Autodesk Inventor part; units mm, degrees
ref_plane "Work Plane1" through (-12.7, 65.9911, 38.1) normal (0, 0.866, 0.5) x (1, 0, 0)
ref_plane "YZ Plane" through (0, 0, 0) normal (1, 0, 0) x (0, 1, 0)
ref_plane "XZ Plane" through (0, 0, 0) normal (0, 1, 0) x (-1, 0, 0)
sketch "Sketch1" plane through (0, 0, 0) normal (1, 0, 0) x (0, 1, 0)
  line L0 (0, 0) -> (0, -762)
  line L1 (0, -762) -> (439.9409, -762)
  line L2 (439.9409, -762) -> (0, 0)
  line L3 (25.4, -129.7892) -> (25.4, -736.6)
  line L4 (25.4, -736.6) -> (361.7607, -736.6)
  line L5 (361.7607, -736.6) -> (25.4, -129.7892)
  dimension "d0" = 762
  dimension "d5" = 30
  dimension "d6" = 1
  dimension "d7" = 25.4
  dimension "d8" = 25.4
extrude "Extrusion1" add sketch "Sketch1" along normal mid plane 25.4 contours L2 L1 L0 | L5 L4 L3
ref_plane "Work Plane1" through (-12.7, 65.9911, 38.1) normal (0, 0.866, 0.5) x (1, 0, 0)
sketch "Sketch3" plane through (12.7, 0, 0) normal (1, 0, 0) x (0, 0, -1)
  line L0 (0, 63.5) -> (873.76, 63.5)
  line L1 (204.7793, 88.9) -> (736.6, 88.9)
  line L2 (736.6, 88.9) -> (736.6, 395.9468)
  line L3 (736.6, 395.9468) -> (204.7793, 88.9)
  line L4 (762, 439.9409) -> (0, 0)
  line L5 (762, 0) -> (762, 439.9409)
  line L6 (0, 0) -> (762, 0)
  line L7 (50.8, 0) -> (160.7852, 63.5)
  line L8 (160.7852, 63.5) -> (762, 63.5)
  line L9 (762, 0) -> (50.8, 0)
  dimension "d14" = 25.4
  dimension "d15" = 25.4
  dimension "d21" = 25.4
extrude "Extrusion4" cut sketch "Sketch3" against normal through all contours L0 L5 L6 L7 | L3 L2 L1
properties part number "ballSupport" material "Aluminum 6061, Welded"
Work out the finished part from the listing and answer in its coordinate system (mm). A direction names the side the tool comes from. Coordinates: 2 decimals unless noted, no trailing zeros. Loops run counter-clockwise (first coordinate to the right, second up) from the corner with the lowest first, then second, coordinate; pieces in that order, holes last. Notation, with made-up numbers: M 20.5,37.5 L 65.5,37.5 A33 cw 65.5,66.5 Z; hole C 55.5,81 d3. An arc over 180 degrees is marked long. Use CSV: the item, a comma, the result in double quotes. Start each with the question number.
(1) Find section C-C, the plane y = 370.5. Give the vertices of the cut face in (x, z), then the cut area to 3 significant figures.
(2) Consider line 1 (Y direction, x = 8.5, z = -545); line 2 (Z direction, x = 7.75, y = 395.5); line 3 (Z direction, x = -1.75, y = 254). Determine where each line is inside the solid, lowest interval first.
(3) Find section A-A, the plane x = -4.5. Give the vertices of the cut face in (y, z).
(4) Given pin 1 Ø4 at (x, y) = (-4.5, 341) entering from +Z; pin 2 Ø1.5 at (x, z) = (-4.5, -354) entering from +Y (3 decimals); pin 3 Ø10 at (x, z) = (8, -288.5) entering from +Y, each flat-ended and moving along its own axis, determine where each tip first touches the part or whether it passes through.
(5) For faces 1 (the face through (0, 63.5, -457)), 2 (the face through (0, 249, -762)), 3 (the face through (0, 240, -736.6)), determine the directions among +Z, -Z, +X, -X, +Y, -Y from which every point of the face is accessible in a straight line to the end or side of a thin tool.
(6) Find section D-D, the plane z = -142. Give the vertices of the cut face in (x, y), then the cut area to 3 significant figures.
(7) Find section B-B, the plane z = -378.5. Give the vertices of the cut face in (x, y).
(8) For a pull along Y with two mould halves and no side action, classify faces 4 (the face through (0, 88.9, -467)), 5 (the face through (0.18, 244.57, -474.41)), 6 (the face through (12.7, 88.6, -520.3)), 7 (the face through (0, 0, -25)) as +Y half, -Y half, draft (parallel to the pull), parting line (faces both ways), or undercut.
Recorded:
1,outline,"M -12.7,-762 L 12.7,-762 L 12.7,-736.6 L -12.7,-736.6 Z; M -12.7,-692.52 L 12.7,-692.52 L 12.7,-641.72 L -12.7,-641.72 Z"
1,area,"1,940 mm^2"
2,line 1,"y = 63.5 to 88.9, 285.33 to 314.66"
2,line 2,"z = -762 to -736.6, -735.83 to -685.03"
2,line 3,"z = -762 to -736.6, -490.74 to -439.94"
3,outline,"M 0,-50.8 L 63.5,-160.79 L 63.5,-762 L 439.94,-762 L 0,0 Z; hole M 88.9,-736.6 L 395.95,-736.6 L 88.9,-204.78 Z"
4,pin 1,"stops at z = -587.17"
4,pin 2,"stops at y = 204.815"
4,pin 3,"stops at y = 169.45"
5,face 1,"-Z, +X, -X, -Y"
5,face 2,"-Z, +X, -X, +Y, -Y"
5,face 3,"+X, -X"
6,outline,"M -12.7,52.65 L 12.7,52.65 L 12.7,81.98 L -12.7,81.98 Z"
6,area,"745 mm^2"
7,outline,"M -12.7,63.5 L 12.7,63.5 L 12.7,88.9 L -12.7,88.9 Z; M -12.7,189.2 L 12.7,189.2 L 12.7,218.53 L -12.7,218.53 Z"
8,face 4,"undercut"
8,face 5,"undercut"
8,face 6,"draft"
8,face 7,"-Y half"
